The model under review builds one solid part; all positions refer to its coordinate system, in mm. A direction names the side the tool comes from. Round coordinates to 2 decimals unless told otherwise and drop trailing zeros. Loops run counter-clockwise (first coordinate to the right, second up) from the corner with the lowest first, then second, coordinate; pieces in that order, holes last. Notation, with made-up numbers: (1.25, -16) -> (32.25, -16) arc R17 cw to (32.25, 15) -> close; hole circle Ø2 at (-20.75, 34). An arc over 180 degrees is marked (long way). Return JSON: item names as keys, results as strings. Group by question number.
```python
from build123d import *

# Parameters (mm, degrees)
SKETCH1_W                                      = 64
SKETCH1_H                                      = 24
BOSS_EXTRUDE1_DEPTH                            = 1.5
SKETCH2_W                                      = 40
SKETCH2_H                                      = 8
CUT_EXTRUDE1_DEPTH                             = 35.208916966
FILLET1_R                                      = 3
CSK_FOR_M2_5_FLAT_HEAD_MACHINE_SCREW1_AT_COUNT = 2
CSK_FOR_M2_5_FLAT_HEAD_MACHINE_SCREW1_AT_PITCH = 58
CSK_FOR_M2_5_FLAT_HEAD_MACHINE_SCREW_2_COUNT   = 2
CSK_FOR_M2_5_FLAT_HEAD_MACHINE_SCREW_2_PITCH   = 18
CSK_FOR_M2_5_FLAT_HEAD_MACHINE_SCREW_3_COUNT   = 2
CSK_FOR_M2_5_FLAT_HEAD_MACHINE_SCREW_3_PITCH   = 60.728905803


with BuildPart() as part:
    # Sketch1 → Boss-Extrude1 (new body)
    with BuildSketch(Plane.XY):
        Rectangle(SKETCH1_W, SKETCH1_H)
    extrude(amount=-BOSS_EXTRUDE1_DEPTH)

    # Sketch2 → Cut-Extrude1 (cut, through all)
    with BuildSketch(Plane.XY):
        with Locations((0, -1.5)):
            Rectangle(SKETCH2_W, SKETCH2_H)
    extrude(amount=-CUT_EXTRUDE1_DEPTH, mode=Mode.SUBTRACT)

    # Fillet1
    fillet1_edges = [part.edges().sort_by_distance(p)[0] for p in [
        (-32, 12, -0.75),
        (32, 12, -0.75),
    ]]
    fillet(fillet1_edges, radius=FILLET1_R)

    # Sketch3 → CSK for M2.5 Flat Head Machine Screw1 (revolve, cut)
    with BuildSketch(Plane(origin=(-29, 9, 0), x_dir=(0, -1, 0), z_dir=(1, 0, 0))):
        Polygon((0, 0), (0, 1.5), (1.45, 1.5), (1.45, 1.3), (2.75, 0), align=None)
    csk_for_m2_5_flat_head_machine_screw1 = revolve(axis=Axis((-29, 9, 6.35), (0, 0, -1)), mode=Mode.SUBTRACT)

    # CSK for M2.5 Flat Head Machine Screw1 at: CSK for M2.5 Flat Head Machine Screw1 ×2
    with Locations(*[(i * CSK_FOR_M2_5_FLAT_HEAD_MACHINE_SCREW1_AT_PITCH, 0, 0) for i in range(1, CSK_FOR_M2_5_FLAT_HEAD_MACHINE_SCREW1_AT_COUNT)]):
        add(csk_for_m2_5_flat_head_machine_screw1, mode=Mode.SUBTRACT)

    # CSK for M2.5 Flat Head Machine Screw 2: CSK for M2.5 Flat Head Machine Screw1 ×2
    with Locations(*[(0, -i * CSK_FOR_M2_5_FLAT_HEAD_MACHINE_SCREW_2_PITCH, 0) for i in range(1, CSK_FOR_M2_5_FLAT_HEAD_MACHINE_SCREW_2_COUNT)]):
        add(csk_for_m2_5_flat_head_machine_screw1, mode=Mode.SUBTRACT)

    # CSK for M2.5 Flat Head Machine Screw 3: CSK for M2.5 Flat Head Machine Screw1 ×2
    with Locations(*[Vector(0.9550641368112371, -0.29639921487245297, 0) * (i * CSK_FOR_M2_5_FLAT_HEAD_MACHINE_SCREW_3_PITCH) for i in range(1, CSK_FOR_M2_5_FLAT_HEAD_MACHINE_SCREW_3_COUNT)]):
        add(csk_for_m2_5_flat_head_machine_screw1, mode=Mode.SUBTRACT)


solid = part.part
```
1. We need section C-C, the plane x = -16. Write out the cut boundary in (y, z).
2. We need section A-A, the plane y = -2.25. Write out the cut boundary in (x, z), then the cut area to 3 significant figures.
3. We need section B-B, the plane z = -0.65. Write out the cut boundary in (x, y), then the cut area to 3 significant figures.
4. Tool access review of faces 1 (the face through (-20, -2, -1)), 2 (the face through (0, 12, -1)): name each direction out of +Z, -Z, +X, -X, +Y, -Y from which nothing blocks a thin tool from reaching the whole face with its end or side.
5. For P1, Ø6, axis at x = 0, y = -8.5, coming from the +Z side; P2, Ø4.5, axis at x = -29, y = 9, coming from the +Z side; P3, Ø2.5, axis at x = -29, y = -9, coming from the +Z side, all flat-tipped, find the tip position at first contact; note any pin that passes through.
6. Wall thickness on line 1 (X direction, y = -9, z = -1.4); line 2 (Y direction, x = -29, z = -1.35); line 3 (Y direction, x = -5, z = -0.1): over which ranges is each line inside the solid? List them lowest first.
7. Draft analysis for pull direction Y (two halves, no side actions). For faces 3 (the face through (0, 2.5, -1)), 4 (the face through (31.1, 11.14, -0.76)), 5 (the face through (32, -2, -1)), state which applies: pulls with the +Y half, pulls with the -Y half, needs draft (parallel to the pull), parting line crosses it, or undercut.
Check sheet entries:
{
 "1": {"outline": "(-12, -1.5) -> (-5.5, -1.5) -> (-5.5, 0) -> (-12, 0) -> close; (2.5, -1.5) -> (12, -1.5) -> (12, 0) -> (2.5, 0) -> close"},
 "2": {"outline": "(-32, -1.5) -> (-20, -1.5) -> (-20, 0) -> (-32, 0) -> close; (20, -1.5) -> (32, -1.5) -> (32, 0) -> (20, 0) -> close", "area": "36.0 mm²"},
 "3": {"outline": "(-32, -12) -> (32, -12) -> (32, 9) arc R3 ccw to (29, 12) -> (-29, 12) arc R3 ccw to (-32, 9) -> close; hole circle Ø4.2 at (-29, -9); hole circle Ø4.2 at (-29, 9); hole (-20, -5.5) -> (20, -5.5) -> (20, 2.5) -> (-20, 2.5) -> close; hole circle Ø4.2 at (29, -9); hole circle Ø4.2 at (29, 9)", "area": "1,160 mm²"},
 "4": {"face 1": "+Z, -Z", "face 2": "+Z, -Z, +X, -X, +Y"},
 "5": {"P1": "stops at z = 0", "P2": "stops at z = -0.5", "P3": "passes through"},
 "6": {"line 1": "x = -32 to -30.45, -27.55 to 27.55, 30.45 to 32", "line 2": "y = -12 to -10.45, -7.55 to 7.55, 10.45 to 12", "line 3": "y = -12 to -5.5, 2.5 to 12"},
 "7": {"face 3": "undercut", "face 4": "pulls with the +Y half", "face 5": "needs draft"}
}
